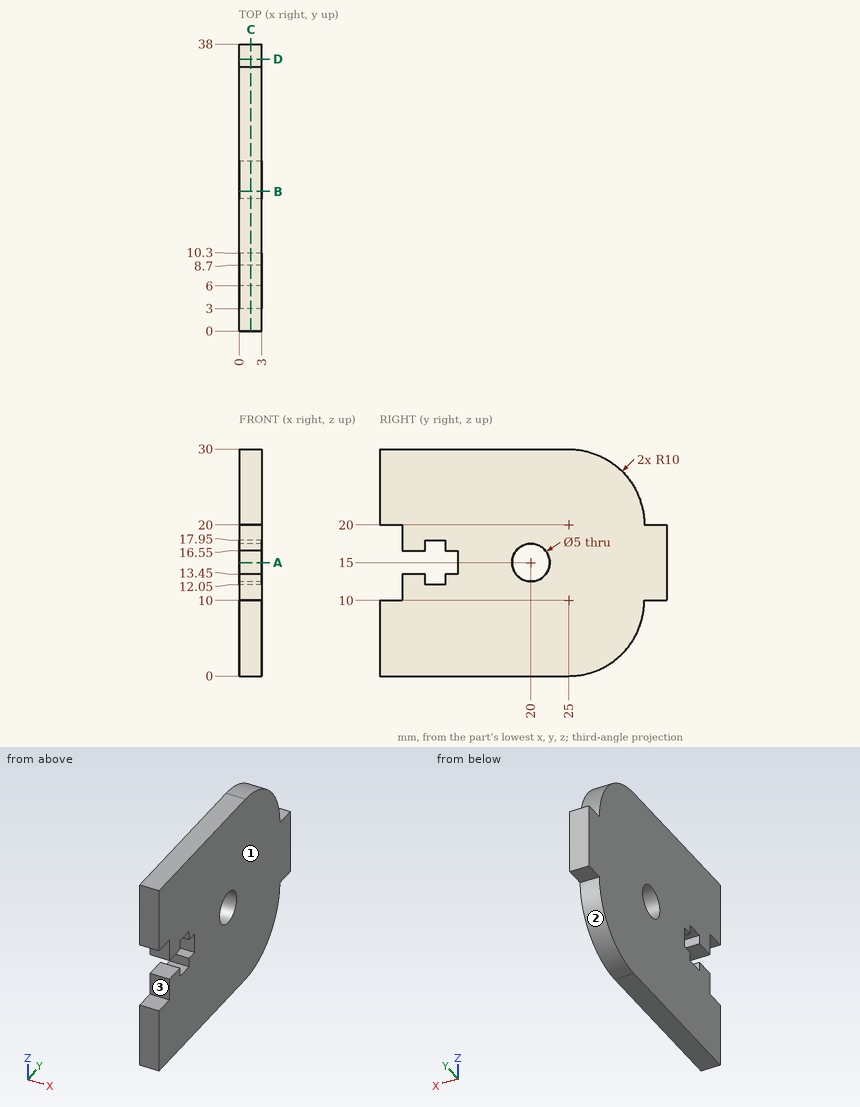
Can you work these out from the drawing? Everything is in mm from the part's minimum corner. Coordinates: 2 decimals unless noted, no trailing zeros. Loops run counter-clockwise (first coordinate to the right, second up) from the corner with the lowest first, then second, coordinate; pieces in that order, holes last. Notation, with made-up numbers: (54, 71) - (109, 71) arc R28 cw to (109, 109) - close; hole circle Ø11 at (46.25, -1). An arc over 180 degrees is marked (long way). Use a Markdown table: item, result.
Item 1: I want a section at D-D on y = 36. Please give me the cut outline in (x, z).
Numbers:
| item | result |
|---|---|
| outline | (0, 10) - (3, 10) - (3, 20) - (0, 20) - close |
Item 2: Will these pins go through, and if not, where does the flat tip stop? pin 1 (2 mm diameter, centred on y = 32.5, z = 25, fed in from -X); pin 2 (4 mm diameter, centred on y = 20, z = 15, fed in from +X); pin 3 (0.9 mm diameter, centred on x = 2, y = 36.5, fed in from -Z); pin 4 (0.7 mm diameter, centred on x = 1.5, z = 12.5, fed in from -Y).
Numbers:
| item | result |
|---|---|
| pin 1 | stops at x = 0 |
| pin 2 | passes through |
| pin 3 | stops at z = 10 |
| pin 4 | stops at y = 3 |
Item 3: I want a section at B-B on y = 18.5. Please give me the cut outline in (x, z), and give its area (3 significant figures).
Numbers:
| item | result |
|---|---|
| outline | (0, 0) - (3, 0) - (3, 13) - (0, 13) - close; (0, 17) - (3, 17) - (3, 30) - (0, 30) - close |
| area | 78.0 mm2 |
Item 4: If I drill on probe 1 along Y at (x, z) = (0.7, 15); probe 2 along Z at (x, y) = (1.3, 9); probe 3 along Z at (x, y) = (1.75, 20), over which ranges is the centre line in solid material (lowest first)? Write a range as from..to.
Numbers:
| item | result |
|---|---|
| probe 1 | y = 10.3..17.5, 22.5..38 |
| probe 2 | z = 0..13.45, 16.55..30 |
| probe 3 | z = 0..12.5, 17.5..30 |
Item 5: I want a section at A-A on z = 15. Please give me the cut outline in (x, y), and give its area (3 significant figures).
Numbers:
| item | result |
|---|---|
| outline | (0, 10.3) - (3, 10.3) - (3, 17.5) - (0, 17.5) - close; (0, 22.5) - (3, 22.5) - (3, 38) - (0, 38) - close |
| area | 68.1 mm2 |
Item 6: I want a section at C-C on x = 1.55. Please give me the cut outline in (y, z), and give its area (3 significant figures).
Numbers:
| item | result |
|---|---|
| outline | (0, 0) - (25, 0) arc R10 ccw to (35, 10) - (38, 10) - (38, 20) - (35, 20) arc R10 ccw to (25, 30) - (0, 30) - (0, 20) - (3, 20) - (3, 16.55) - (6, 16.55) - (6, 17.95) - (8.7, 17.95) - (8.7, 16.55) - (10.3, 16.55) - (10.3, 13.45) - (8.7, 13.45) - (8.7, 12.05) - (6, 12.05) - (6, 13.45) - (3, 13.45) - (3, 10) - (0, 10) - close; hole circle Ø5 at (20, 15) |
| area | 957 mm2 |
Item 7: We'd pull the mould along Z, two halves only. Please class the marked faces 1, 2 and 3: released by +Z, released by -Z, zero draft, split by the parting line, or undercut.
Numbers:
| item | result |
|---|---|
| face 1 | zero draft |
| face 2 | released by -Z |
| face 3 | undercut |
